from build123d import *

# Parameters (mm, degrees)
SKETCH1_W              = 278.607499934
SKETCH1_H              = 496.8875
BOSS_EXTRUDE1_DEPTH    = 157.48
CONVERT_SOLID1_START   = -152.826113143
CONVERT_SOLID1_DEPTH   = 278.607499934
CONVERT_SOLID1_2_DEPTH = 278.607499934


# Read off the part's stored shape, not the designer's step: Convert-Solid1
with BuildPart() as part:
    # Sketch1 → Boss-Extrude1 (new body)
    with BuildSketch(Plane.XY):
        with Locations((-13.522363176, 152.341784507)):
            Rectangle(SKETCH1_W, SKETCH1_H)
    extrude(amount=BOSS_EXTRUDE1_DEPTH)

    # Convert-Solid1 outline → Convert-Solid1 (cut)
    with BuildSketch(Plane.YZ.offset(CONVERT_SOLID1_START)):
        with BuildLine():
            Line((398.405534441, 157.48), (-96.101965493, 157.48))
            Line((-96.101965493, 157.48), (-96.101965493, 0))
            Line((-96.101965493, 0), (400.785534507, 0))
            Line((400.785534507, 0), (400.785534507, 155.099999934))
            ThreePointArc((400.785534507, 155.099999934), (400.088448627, 156.78291412), (398.405534441, 157.48))
        make_face()
    extrude(amount=CONVERT_SOLID1_DEPTH, mode=Mode.SUBTRACT)

    # Convert-Solid1 2 outline → Convert-Solid1 2 (add)
    with BuildSketch(Plane.YZ.offset(CONVERT_SOLID1_START)):
        with BuildLine():
            Line((398.405534441, 159.0675), (-96.101965493, 159.0675))
            Line((-96.101965493, 159.0675), (-96.101965493, 157.48))
            Line((-96.101965493, 157.48), (400.785534507, 157.48))
            Line((400.785534507, 157.48), (400.785534507, 0))
            Line((400.785534507, 0), (402.373034507, 0))
            Line((402.373034507, 0), (402.373034507, 155.099999934))
            ThreePointArc((402.373034507, 155.099999934), (401.210980642, 157.905446136), (398.405534441, 159.0675))
        make_face()
    extrude(amount=CONVERT_SOLID1_2_DEPTH)


solid = part.part
For this review, take the finished solid that the model builds, in its own axes (mm). A direction names the side the tool comes from. Round coordinates to 2 decimals unless told otherwise and drop trailing zeros. Order: outer loops, then holes, each group sorted by start corner. A loop starts at its lowest first (then second) coordinate and runs counter-clockwise, first axis right, second up. Notation, with made-up numbers: M 34,77 L 81,77 A10 ccw 81,85 Z; hole C 21,-20 d2. An arc over 180 degrees is marked long. Write each question's results on one line, items separated by ' | '. Start each with the question number.
1. Clearance check with flat-ended pins moving along their axes: pin 1 Ø1.5 at (x, y) = (39, 341) entering from -Z; pin 2 Ø10 at (x, z) = (-50, 26.5) entering from -Y. State where each tip first meets the part, or that it passes through.
2. Add section A-A (x = -27). State the section outline as (y, z) points (1 decimal), then the cut area to 3 significant figures.
3. Tool access review of faces 1 (the face through (-15, 402.373, 76)), 2 (the face through (-15, 148, 157.48)): name each direction out of +Z, -Z, +X, -X, +Y, -Y from which nothing blocks a thin tool from reaching the whole face with its end or side.
4. Add section C-C (z = 90). State the section outline as (x, y) points.
5. To check wall thickness, follow L1, parallel to Y at x = 77, z = 64; L2, parallel to Z at x = 18, y = 94.5. State the ranges of each line that lie inside material, in increasing order. Write a range as [from, to].
6. Add section B-B (y = 133). State the section outline as (x, z) points.
Output values:
1) pin 1: z = 157.48 | pin 2: y = 400.79
2) outline: M -96.1,157.5 L 398.4,157.5 A2.4 cw 400.8,155.1 L 400.8,0 L 402.4,0 L 402.4,155.1 A4 ccw 398.4,159.1 L -96.1,159.1 Z | area: 1,040 mm^2
3) face 1: +Z, -Z, +X, -X, +Y | face 2: -Z, +X, -X, -Y
4) outline: M -152.83,400.79 L 125.78,400.79 L 125.78,402.37 L -152.83,402.37 Z
5) L1: [400.79, 402.37] | L2: [157.48, 159.07]
6) outline: M -152.83,157.48 L 125.78,157.48 L 125.78,159.07 L -152.83,159.07 Z
